Geometry: final body of the model. Coordinates: model frame, mm. A direction names the side the tool comes from. Coordinates: 2 decimals unless noted, no trailing zeros. Order: outer loops, then holes, each group sorted by start corner. A loop starts at its lowest first (then second) coordinate and runs counter-clockwise, first axis right, second up. Notation, with made-up numbers: M 53,55 L 94,55 A26 cw 94,74 Z; hole C 46.25,-5.5 d5. An arc over 180 degrees is marked long. Use CSV: the item, a comma, the result in double quotes. Start each with the question number.
1. Section query B-B on z = 25.5. Return the cut outline in (x, y).
2. First-contact query: P1, Ø1, axis at y = -5, z = 29, coming from the -X side; P2, Ø6, axis at y = -10.5, z = 7.5, coming from the +X side; P3, Ø6.5, axis at y = 38, z = -3.5, coming from the -X side; P4, Ø1.5, axis at y = -18, z = 5, coming from the +X side. Flat tips, straight axial feed; report the tip coordinate or a pass-through.
3. Section query A-A on x = 17. Return the cut outline in (y, z).
4. Section query C-C on y = -54. State how many separate pieces and enclosed holes the cut face has, and give its area (3 significant figures).
5. Section query D-D on x = -35. Return the cut outline in (y, z).
6. Material intervals for line 1 (X direction, y = -40, z = -0.5); line 2 (X direction, y = -10.5, z = 1); line 3 (Z direction, x = 10.45, y = -8.8), sorted ascending.
7. Set-up query: faces 1 (the cylindrical face through (10.314, -9.944, 32.513)), 2 (the flat face through (-3.5, -37, -3)), 3 (the cylindrical face through (0.1, 28.5, -3)). Return all of +Z, -Z, +X, -X, +Y, -Y with unobstructed straight access to the full face (end or side cutting, diameter ignored); none if empty.
from build123d import *

# Parameters (mm, degrees)
SKETCH_W             = 18.6
SKETCH_H             = 93
PAD_DEPTH            = 6
SKETCH001_W          = 3
SKETCH001_H          = 6
POCKET_DEPTH         = 6
POCKET001_DEPTH      = 8
PAD001_DEPTH         = 2
SKETCH004_R          = 1.551846
SKETCH004_R_2        = 1.552141
POCKET002_DEPTH      = 20.601
SKETCH005_W          = 80
SKETCH005_H          = 40
PAD002_DEPTH         = 2
POCKET003_DEPTH      = 5
LINEARPATTERN_COUNT  = 8
LINEARPATTERN_PITCH  = 11.428571
SKETCH007_W          = 80
SKETCH007_H          = 40
PAD003_DEPTH         = 2.2
POCKET004_DEPTH      = 5
SKETCH009_R          = 5.6651
SKETCH009_R_2        = 1.478967
POCKET005_DEPTH      = 15
POCKET005_DEPTH_BACK = -15


with BuildPart() as part:
    # Sketch → Pad (new body)
    with BuildSketch(Plane.XY):
        Rectangle(SKETCH_W, SKETCH_H)
    extrude(amount=-PAD_DEPTH)

    # Sketch001 (on Face5 of Pad) → Pocket (cut)
    with BuildSketch(Plane.XY):
        Rectangle(SKETCH001_W, SKETCH001_H)
    extrude(amount=-POCKET_DEPTH, mode=Mode.SUBTRACT)

    # Sketch002 (on Face4 of Pocket) → Pocket001 (cut)
    with BuildSketch(Plane.XY):
        with BuildLine():
            ThreePointArc((-2.5, -42), (0, -44.5), (2.5, -42))
            Line((2.5, -42), (2.5, -32))
            ThreePointArc((2.5, -32), (0, -29.5), (-2.5, -32))
            Line((-2.5, -42), (-2.5, -32))
        make_face()
        with BuildLine():
            ThreePointArc((-8.5, -42), (-6, -44.5), (-3.5, -42))
            Line((-3.5, -42), (-3.5, -32))
            ThreePointArc((-3.5, -32), (-6, -29.5), (-8.5, -32))
            Line((-8.5, -42), (-8.5, -32))
        make_face()
        with BuildLine():
            ThreePointArc((3.5, -42), (6, -44.5), (8.5, -42))
            Line((8.5, -42), (8.5, -32))
            ThreePointArc((8.5, -32), (6, -29.5), (3.5, -32))
            Line((3.5, -42), (3.5, -32))
        make_face()
        with BuildLine():
            ThreePointArc((-2.487782, -26), (0.012218, -28.5), (2.512218, -26))
            Line((2.512218, -26), (2.512218, -16))
            ThreePointArc((2.512218, -16), (0.012218, -13.5), (-2.487782, -16))
            Line((-2.487782, -26), (-2.487782, -16))
        make_face()
        with BuildLine():
            ThreePointArc((-8.496945, -26), (-6, -28.496945), (-3.503055, -26))
            Line((-3.503055, -26), (-3.503055, 8))
            ThreePointArc((-3.503055, 8), (-6, 10.496945), (-8.496945, 8))
            Line((-8.496945, -26), (-8.496945, 8))
        make_face()
        with BuildLine():
            ThreePointArc((3.503055, -26), (6, -28.496945), (8.496945, -26))
            Line((8.496945, -26), (8.496945, 8))
            ThreePointArc((8.496945, 8), (6, 10.496945), (3.503055, 8))
            Line((3.503055, -26), (3.503055, 8))
        make_face()
        with BuildLine():
            ThreePointArc((2.5, 42), (0, 44.5), (-2.5, 42))
            Line((-2.5, 42), (-2.5, 32))
            ThreePointArc((-2.5, 32), (0, 29.5), (2.5, 32))
            Line((2.5, 42), (2.5, 32))
        make_face()
        with BuildLine():
            ThreePointArc((-3.5, 42), (-6, 44.5), (-8.5, 42))
            Line((-8.5, 42), (-8.5, 32))
            ThreePointArc((-8.5, 32), (-6, 29.5), (-3.5, 32))
            Line((-3.5, 42), (-3.5, 32))
        make_face()
        with BuildLine():
            ThreePointArc((8.5, 42), (6, 44.5), (3.5, 42))
            Line((3.5, 42), (3.5, 32))
            ThreePointArc((3.5, 32), (6, 29.5), (8.5, 32))
            Line((8.5, 42), (8.5, 32))
        make_face()
        with BuildLine():
            ThreePointArc((2.512218, 26), (0.012218, 28.5), (-2.487782, 26))
            Line((-2.487782, 26), (-2.487782, 16))
            ThreePointArc((-2.487782, 16), (0.012218, 13.5), (2.512218, 16))
            Line((2.512218, 26), (2.512218, 16))
        make_face()
        with BuildLine():
            ThreePointArc((-3.487782, 26), (-5.987782, 28.5), (-8.487782, 26))
            Line((-8.487782, 26), (-8.487782, 16))
            ThreePointArc((-8.487782, 16), (-5.987782, 13.5), (-3.487782, 16))
            Line((-3.487782, 26), (-3.487782, 16))
        make_face()
        with BuildLine():
            ThreePointArc((8.496945, 26), (6, 28.496945), (3.503055, 26))
            Line((3.503055, 26), (3.503055, 16))
            ThreePointArc((3.503055, 16), (6, 13.503055), (8.496945, 16))
            Line((8.496945, 26), (8.496945, 16))
        make_face()
    extrude(amount=-POCKET001_DEPTH, mode=Mode.SUBTRACT)

    # Sketch003 (on Face3 of Pocket001) → Pad001 (join)
    with BuildSketch(Plane.YZ.offset(9.3)):
        Polygon((-24, -6), (-24, 0), (-10.960923, 6), (-10.960923, 37), (-3, 37), (-3, 6), (3, 6), (3, 37), (10.971753, 37), (10.971753, 6), (24, 0), (24, -6), align=None)
    pad001 = extrude(amount=PAD001_DEPTH)

    # Sketch004 → Pocket002 (cut, through all)
    with BuildSketch(Plane.YZ.offset(11.3)):
        with Locations((-8.8, 31.464135)):
            Circle(SKETCH004_R)
        with Locations((8.8, 31.541361)):
            Circle(SKETCH004_R_2)
    extrude(amount=-POCKET002_DEPTH, mode=Mode.SUBTRACT)

    # Sketch005 (on Face5 of Pocket002) → Pad002 (join)
    with BuildSketch(Plane(origin=(0, 0, -6), x_dir=(1, 0, 0), z_dir=(0, 0, -1))):
        with Locations((0, 60)):
            Rectangle(SKETCH005_W, SKETCH005_H)
    extrude(amount=-PAD002_DEPTH)

    # Sketch006 (on Face66 of Pad002) → Pocket003 (cut)
    with BuildSketch(Plane(origin=(0, 0, -6), x_dir=(1, 0, 0), z_dir=(0, 0, -1))):
        with BuildLine():
            ThreePointArc((-31.836483, 75), (-35, 78.163517), (-38.163517, 75))
            Line((-38.163517, 75), (-38.163517, 45))
            ThreePointArc((-38.163517, 45), (-35, 41.836483), (-31.836483, 45))
            Line((-31.836483, 75), (-31.836483, 45))
        make_face()
    pocket003 = extrude(amount=-POCKET003_DEPTH, mode=Mode.SUBTRACT)

    # LinearPattern: Pocket003 ×8
    with Locations(*[(i * LINEARPATTERN_PITCH, 0, 0) for i in range(1, LINEARPATTERN_COUNT)]):
        add(pocket003, mode=Mode.SUBTRACT)

    # Sketch007 (on Face5 of LinearPattern) → Pad003 (join)
    with BuildSketch(Plane(origin=(0, 0, -6), x_dir=(1, 0, 0), z_dir=(0, 0, -1))):
        with Locations((0, -60)):
            Rectangle(SKETCH007_W, SKETCH007_H)
    extrude(amount=-PAD003_DEPTH)

    # Sketch008 (on Face111 of Pad003) → Pocket004 (cut)
    with BuildSketch(Plane(origin=(0, 0, -6), x_dir=(1, 0, 0), z_dir=(0, 0, -1))):
        with BuildLine():
            ThreePointArc((-31.490648, -45), (-35, -41.490648), (-38.509352, -45))
            Line((-38.509352, -45), (-38.509352, -75))
            ThreePointArc((-38.509352, -75), (-35, -78.509352), (-31.490648, -75))
            Line((-31.490648, -45), (-31.490648, -75))
        make_face()
    extrude(amount=-POCKET004_DEPTH, mode=Mode.SUBTRACT)

    # Mirrored: Pad001 across YZ
    add(pad001.mirror(Plane.YZ))

    # Sketch009 → Pocket005 (cut, two sides)
    with BuildSketch(Plane.YZ) as pocket005_sk:
        with Locations((0, 11.65735)):
            Circle(SKETCH009_R)
        with Locations((-8.758097, 31.478674)):
            Circle(SKETCH009_R_2)
    extrude(amount=-POCKET005_DEPTH, mode=Mode.SUBTRACT)
    extrude(pocket005_sk.sketch, amount=-POCKET005_DEPTH_BACK, mode=Mode.SUBTRACT)


solid = part.part
Results list:
1,outline,"M -11.3,-10.96 L -9.3,-10.96 L -9.3,-3 L -11.3,-3 Z; M -11.3,3 L -9.3,3 L -9.3,10.97 L -11.3,10.97 Z; M 9.3,-10.96 L 11.3,-10.96 L 11.3,-3 L 9.3,-3 Z; M 9.3,3 L 11.3,3 L 11.3,10.97 L 9.3,10.97 Z"
2,P1,"stops at x = -11.3"
2,P2,"stops at x = 11.3"
2,P3,"stops at x = -40"
2,P4,"passes through"
3,outline,"M -80,-6 L -40,-6 L -40,-4 L -80,-4 Z; M 40,-6 L 80,-6 L 80,-3.8 L 40,-3.8 Z"
4,separate pieces,"8"
4,enclosed holes,"0"
4,area,"71.4 mm²"
5,outline,"M -80,-6 L -78.16,-6 L -78.16,-4 L -80,-4 Z; M -41.84,-6 L -40,-6 L -40,-4 L -41.84,-4 Z; M 40,-6 L 41.49,-6 L 41.49,-3.8 L 40,-3.8 Z; M 78.51,-6 L 80,-6 L 80,-3.8 L 78.51,-3.8 Z"
6,line 1,"x = -9.3 to -8.5, -3.5 to -2.5, 2.5 to 3.5, 8.5 to 9.3"
6,line 2,"x = -11.3 to -9.3, 9.3 to 11.3"
6,line 3,"z = -6 to 29.91, 33.02 to 37"
7,face 1,"+X"
7,face 2,"+Z"
7,face 3,"+Z, -Z"
